Here's how the part is built. I have some questions about the finished solid (model axes, mm). Face numbers are marked on the shaded views. A direction names the side the tool comes from. Give positions to 0.01 mm unless a question says otherwise; leave off trailing zeros. Loops run counter-clockwise (first coordinate to the right, second up) from the corner with the lowest first, then second, coordinate; pieces in that order, holes last. Notation, with made-up numbers: (-25.5, -35.5) - (-0.5, -35.5) arc R12 cw to (-0.5, -19.5) - close; hole circle Ø1 at (70.25, 45). An arc over 180 degrees is marked (long way). Use a Markdown table: item, result.
Autodesk Inventor part; units mm, degrees
ref_plane "YZ Plane" through (0, 0, 0) normal (1, 0, 0) x (0, 1, 0)
ref_plane "XZ Plane" through (0, 0, 0) normal (0, 1, 0) x (-1, 0, 0)
ref_plane "XY Plane" through (0, 0, 0) normal (0, 0, 1) x (1, 0, 0)
sketch "Skizze1" plane through (0, 0, 0) normal (0, 0, 1) x (1, 0, 0)
  line L0 (-103.8791, 0) -> (60.3442, 0)
  line L1 (0, -106.7819) -> (0, 196.5471)
  line L2 (29.5814, -63.4492) -> (29.5814, 94.1623)
  arc A0 (29.5814, 94.1623) -> (-80.4186, 115.4104) centre (-29.4958, 83.6793) ccw
  line L3 (-80.4186, 115.4104) -> (-10.4186, 86.5508)
  line L4 (-10.4186, 86.5508) -> (9.5814, -63.4492)
  line L5 (9.5814, -63.4492) -> (29.5814, -63.4492)
  point P0 (0, 0)
  point P1 (-57.3059, 105.8815)
  dimension "d0" = 120
  dimension "d2" = 20
  dimension "d3" = 40
  dimension "d4" = 120
  dimension "d6" = 150
  dimension "d24" = 70
extrude "Extrusion1" add sketch "Skizze1" along normal blind 4 contours L4 L1 A0 L2 L0 | L0 L2 L5 L4 | L4 L3 A0 L1
sketch "Skizze2" plane through (0, 0, 4) normal (0, 0, 1) x (1, 0, 0)
  arc A0 (-82.3244, 110.7879) -> (-59.2117, 101.2589) centre (-70.768, 106.0234) ccw
  line L0 (29.5814, -63.4492) -> (29.5814, 94.1623)
  line L1 (9.5814, -63.4492) -> (29.5814, -63.4492)
  point P0 (0, 0)
  point P1 (19.5814, -53.4492)
  dimension "d15" = 10
  dimension "d16" = 10
hole "Bohrung1" at (19.5814, -53.4492, 4) direction (0, 0, -1) diameter 3 end through all
sketch "Skizze3" plane through (-10.4186, 86.5508, 0) normal (-0.3811568, -0.9245104, 0) x (0.9245104, -0.3811568, 0)
  line L0 (34.0793, 4) -> (-75.7158, 4)
  line L1 (-75.7158, 4) -> (-50.7158, 4)
  line L2 (-50.7158, 4) -> (-50.7158, -11)
  line L3 (-50.7158, -11) -> (-75.7158, -11)
  line L4 (-75.7158, -11) -> (-75.7158, 4)
  point P0 (42.6216, 0)
  dimension "d25" = 15
  dimension "d26" = 25
extrude "Extrusion2" add sketch "Skizze3" along normal blind 10
sketch "Skizze4" plane through (-80.4186, 115.4104, -11) normal (-0.9245104, 0.3811568, 0) x (0, 0, 1)
  line L0 (11, 0) -> (11, 50.0739)
  line L1 (0, 0) -> (0, -10)
  line L2 (11, 0) -> (0, 0)
  line L3 (11, 0) -> (15, 0)
  line L4 (0, -10) -> (15, -10)
  line L5 (11, 0) -> (6, -5)
  line L6 (15, 0) -> (15, -10)
  line L7 (15, 0) -> (10, -5)
  line L8 (6, -5) -> (10, -5)
  point P0 (11, -76.046)
  point P1 (11, 22.2831)
  dimension "d30" = 5
  dimension "d31" = 5
  dimension "d32" = 45
extrude "Extrusion3" cut sketch "Skizze4" against normal blind 25 contours L2 L5 L8 L7 L6 L4 L1
sketch "Skizze5" plane through (-82.3244, 110.7879, -5) normal (-0.3811568, -0.9245104, 0) x (0.9245104, -0.3811568, 0)
  point P0 (118.3373, 5)
sketch "Skizze6" plane through (-82.3244, 110.7879, -5) normal (-0.3811568, -0.9245104, 0) x (0.9245104, -0.3811568, 0)
  point P0 (118.3373, 5)
sketch "Skizze7" plane through (-82.3244, 110.7879, -5) normal (-0.3811568, -0.9245104, 0) x (0.9245104, -0.3811568, 0)
  point P0 (118.3373, 5)
sketch "Skizze8" plane through (-82.3244, 110.7879, -5) normal (-0.3811568, -0.9245104, 0) x (0.9245104, -0.3811568, 0)
  line L0 (25, 4) -> (25, 0)
  line L1 (0, 0) -> (25, 0)
  line L2 (25, 0) -> (25, 4)
  line L3 (25, 4) -> (0, 4)
  line L4 (0, 4) -> (0, 0)
  point P0 (118.3373, 5)
  point P1 (25, 0)
extrude "Extrusion4" add sketch "Skizze8" along normal blind 25
sketch "Skizze9" plane through (-91.8533, 87.6751, -1) normal (0, 0, 1) x (0.9245104, -0.3811568, 0)
  arc A0 (0, 12.5) -> (25, 12.5) centre (12.5, 12.5) ccw
  line L0 (0, 25) -> (0, 0)
  line L1 (25, 0) -> (0, 0)
  line L2 (25, 25) -> (25, 0)
  line L3 (25, 12.5) -> (25, 0)
  line L4 (0, 0) -> (0, 12.5)
  point P0 (118.3373, -46.046)
  point P1 (12.5, 0)
  dimension "d37" = 25
  dimension "d38" = 12.5
extrude "Extrusion5" cut sketch "Skizze9" against normal blind 30
sketch "Skizze10" plane through (-82.3244, 110.7879, -1) normal (0, 0, 1) x (0.9245104, -0.3811568, 0)
  arc A0 (0, -12.5) -> (25, -12.5) centre (12.5, -12.5) ccw
  point P0 (118.3373, -71.046)
  point P1 (12.5, -12.5)
  dimension "d41" = 0
  dimension "d42" = 0
hole "Bohrung2" at (-75.5325, 94.467, -1) direction (0, 0, -1) diameter 3 end through all
sketch "Skizze12" plane through (0, 0, 4) normal (0, 0, 1) x (1, 0, 0)
  line L0 (-57.3059, 105.8815) -> (-10.4186, 86.5508)
  line L1 (29.5814, -63.4492) -> (29.5814, 94.1623)
  point P0 (0, 0)
  point P1 (9.5814, 99.9383)
  point P2 (14.5814, 19.9383)
  dimension "d63" = 20
  dimension "d64" = 20
  dimension "d65" = 80
  dimension "d66" = 15
hole "Bohrung4" at (9.5814, 99.9383, 4) at (14.5814, 19.9383, 4) direction (0, 0, -1) diameter 3 end through all
properties part number "Halterung hinten oben"
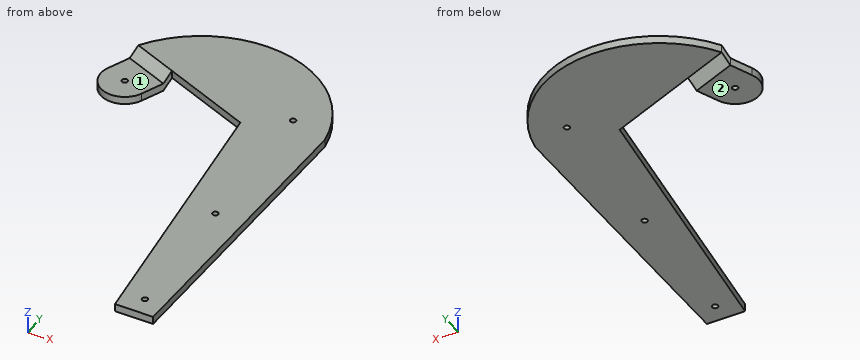
(1) Will these pins go through, and if not, where does the flat tip stop? pin 1 (4 mm diameter, centred on x = 14.58, y = 19.94, fed in from +Z); pin 2 (4 mm diameter, centred on x = -24.5, y = 95.5, fed in from -Z); pin 3 (5 mm diameter, centred on x = -57.5, z = 1, fed in from +Y); pin 4 (3 mm diameter, centred on x = -0.5, z = 3, fed in from +Y).
A:
| item | result |
|---|---|
| pin 1 | z = 4 |
| pin 2 | z = 0 |
| pin 3 | y = 137.99 |
| pin 4 | y = 137.01 |
(2) On a 3-axis mill with a long thin cutter (end or side, diameter ignored), from which of +Z, -Z, +X, -X, +Y, -Y can I reach the whole of each face in a straight line? I mean the marked faces 1 and 2. Say none if no direction works.
A:
| item | result |
|---|---|
| face 1 | +Z, -X, -Y |
| face 2 | -Z, +X, -X, +Y, -Y |
(3) Suppose I cut it at B-B on x = -16. Write out the boundary of the cut face in (y, z).
A:
| item | result |
|---|---|
| outline | (88.85, 0) - (142.14, 0) - (142.14, 4) - (88.85, 4) - close |
(4) Suppose I cut it at C-C on y = 48.5. Write out the boundary of the cut face in (x, z).
A:
| item | result |
|---|---|
| outline | (-5.35, 0) - (29.58, 0) - (29.58, 4) - (-5.35, 4) - close |
(5) Suppose I cut it at A-A on y = 108. Write out the boundary of the cut face in (x, z).
A:
| item | result |
|---|---|
| outline | (-83.47, -5) - (-75.56, -5) - (-62.44, 0) - (25.35, 0) - (25.35, 4) - (-62.44, 4) - (-75.56, -1) - (-83.47, -1) - close |
(6) If I drill on line 1 (Z direction, x = -12.5, y = 109.5); line 2 (Y direction, x = -74.5, z = -4); line 3 (X direction, y = -1, z = 1), over which ranges is the centre line in solid material (lowest first)?
A:
| item | result |
|---|---|
| line 1 | 0 to 4 |
| line 2 | 82.01 to 93.38, 95.56 to 108.64 |
| line 3 | 1.25 to 29.58 |
